```python
from build123d import *

# Parameters (mm, degrees)
CROQUIS1_W                                   = 70
CROQUIS1_H                                   = 30
SALIENTE_EXTRUIR1_DEPTH                      = 3
SALIENTE_EXTRUIR2_DEPTH                      = 24
CORTAR_EXTRUIR1_DEPTH                        = 70.000004
CROQUIS5_R                                   = 1.5
CORTAR_EXTRUIR2_DEPTH                        = 3
REFRENTADO_PARA_TORNILLO_TAP_N_CON_C_2_COUNT = 2
REFRENTADO_PARA_TORNILLO_TAP_N_CON_C_2_PITCH = 30
REFRENTADO_PARA_TORNILLO_TAP_N_CON_C_3_COUNT = 2
REFRENTADO_PARA_TORNILLO_TAP_N_CON_C_3_PITCH = 18.848076825
REFRENTADO_PARA_TORNILLO_TAP_N_CON_C_4_COUNT = 2
REFRENTADO_PARA_TORNILLO_TAP_N_CON_C_4_PITCH = 40.929817982
REDONDEO1_R                                  = 5


with BuildPart() as part:
    # Croquis1 → Saliente-Extruir1 (new body)
    with BuildSketch(Plane.XY):
        with Locations((5.076335878, 0.496183206)):
            Rectangle(CROQUIS1_W, CROQUIS1_H)
    extrude(amount=SALIENTE_EXTRUIR1_DEPTH)

    # Croquis3 → Saliente-Extruir2 (add)
    with BuildSketch(Plane.XY.offset(3)):
        Polygon((-29.923664122, 0.496183206), (40.076335878, 0.496183206), (40.076335878, -4.503816794), (40.076335878, -14.503816794), (36.076335878, -14.503816794), (36.076335878, -4.503816794), (18.076335878, -4.503816794), (18.076335878, -14.503816794), (14.076335878, -14.503816794), (14.076335878, -4.503816794), (-3.923664122, -4.503816794), (-3.923664122, -14.503816794), (-7.923664122, -14.503816794), (-7.923664122, -4.503816794), (-25.923664122, -4.503816794), (-25.923664122, -14.503816794), (-29.923664122, -14.503816794), (-29.923664122, -4.503816794), align=None)
    extrude(amount=SALIENTE_EXTRUIR2_DEPTH)

    # Croquis4 → Cortar-Extruir1 (cut)
    with BuildSketch(Plane.ZY.offset(29.923664122)):
        with BuildLine():
            Line((27, -14.503816794), (27, -4.503816794))
            ThreePointArc((27, -4.503816794), (14.366976751, -7.984560996), (3, -14.503816794))
            Line((3, -14.503816794), (27, -14.503816794))
        make_face()
    extrude(amount=-CORTAR_EXTRUIR1_DEPTH, mode=Mode.SUBTRACT)

    # Croquis5 → Cortar-Extruir2 (cut)
    with BuildSketch(Plane.XY.offset(3)):
        with Locations((-9.923664122, 7.996183206)):
            Circle(CROQUIS5_R)
        with Locations(Location((20.076335878, 7.996183206, 0), (0, 0, 180))):
            Circle(CROQUIS5_R)
        with Locations((-16.923664122, -9.503816794)):
            Circle(CROQUIS5_R)
        with Locations(Location((27.076335878, -9.503816794, 0), (0, 0, 180))):
            Circle(CROQUIS5_R)
    extrude(amount=-CORTAR_EXTRUIR2_DEPTH, mode=Mode.SUBTRACT)

    # Croquis7 → Refrentado para tornillo tapón con cabeza plana de clavija de M31 (revolve, cut)
    with BuildSketch(Plane(origin=(-9.923664122, 7.996183206, 3), x_dir=(0, -1, 0), z_dir=(1, 0, 0))):
        Polygon((0, 0), (0, 3), (1.7, 3), (1.7, 1.66), (3.36, 0), align=None)
    refrentado_para_tornillo_tap_n_con_cabez = revolve(axis=Axis((-9.923664122, 7.996183206, 9.35), (0, 0, -1)), mode=Mode.SUBTRACT)

    # Refrentado para tornillo tap_n con c 2: Refrentado para tornillo tapón con cabeza plana de clavija de M31 ×2
    with Locations(*[(i * REFRENTADO_PARA_TORNILLO_TAP_N_CON_C_2_PITCH, 0, 0) for i in range(1, REFRENTADO_PARA_TORNILLO_TAP_N_CON_C_2_COUNT)]):
        add(refrentado_para_tornillo_tap_n_con_cabez, mode=Mode.SUBTRACT)

    # Refrentado para tornillo tap_n con c 3: Refrentado para tornillo tapón con cabeza plana de clavija de M31 ×2
    with Locations(*[Vector(-0.3713906763541037, -0.9284766908852593, 0) * (i * REFRENTADO_PARA_TORNILLO_TAP_N_CON_C_3_PITCH) for i in range(1, REFRENTADO_PARA_TORNILLO_TAP_N_CON_C_3_COUNT)]):
        add(refrentado_para_tornillo_tap_n_con_cabez, mode=Mode.SUBTRACT)

    # Refrentado para tornillo tap_n con c 4: Refrentado para tornillo tapón con cabeza plana de clavija de M31 ×2
    with Locations(*[Vector(0.9039864290798859, -0.42756114888913443, 0) * (i * REFRENTADO_PARA_TORNILLO_TAP_N_CON_C_4_PITCH) for i in range(1, REFRENTADO_PARA_TORNILLO_TAP_N_CON_C_4_COUNT)]):
        add(refrentado_para_tornillo_tap_n_con_cabez, mode=Mode.SUBTRACT)

    # Redondeo1
    # the kernel refuses this fillet: 5 mm, written as the material it takes off along each edge
    with BuildSketch(Plane(origin=(40.076335878, -14.503816794, 15.5), x_dir=(0, 1, 0), z_dir=(0, 0, -1)), Plane(origin=(-29.923664122, -14.503816794, -12.5), x_dir=(0, 1, 0), z_dir=(0, 0, 1)), Plane(origin=(-29.923664122, 15.496183206, -12.5), x_dir=(1, 0, 0), z_dir=(0, 0, 1))) as redondeo1_piece_1:
        with BuildLine():
            CenterArc((REDONDEO1_R, -REDONDEO1_R), REDONDEO1_R, 90, 90)
            Line((0, -REDONDEO1_R), (0, 0))
            Line((0, 0), (REDONDEO1_R, 0))
        make_face()
    extrude(amount=28, mode=Mode.SUBTRACT)
    with BuildSketch(Plane(origin=(40.076335878, 15.496183206, -12.5), x_dir=(-1, 0, 0), z_dir=(0, 0, 1))) as redondeo1_piece_2:
        with BuildLine():
            CenterArc((REDONDEO1_R, REDONDEO1_R), REDONDEO1_R, 180, 90)
            Line((0, REDONDEO1_R), (0, 0))
            Line((0, 0), (REDONDEO1_R, 0))
        make_face()
    extrude(amount=28, mode=Mode.SUBTRACT)


solid = part.part
```
Verification items for the finished model (mm, model axes). A direction names the side the tool comes from. Coordinates: 2 decimals unless noted, no trailing zeros. Loops run counter-clockwise (first coordinate to the right, second up) from the corner with the lowest first, then second, coordinate; pieces in that order, holes last. Notation, with made-up numbers: (15.25, 55) -> (69.25, 55) arc R27 ccw to (69.25, 94) -> close; hole circle Ø8 at (-25.75, 10). An arc over 180 degrees is marked (long way). Put each result on its own line as item: value.
1. Mould release check, pull along Y, two halves, no side actions. Record for faces 4 (the face through (5, 15.496, 1)), 5 (the face through (14.076, -7, 9)), 6 (the face through (5, -14.504, 1)), 7 (the face through (28.736, -9.135, 0.679)): pulls with the +Y half, pulls with the -Y half, needs draft (parallel to the pull), parting line crosses it, or undercut.
Result set:
face 4: pulls with the +Y half
face 5: needs draft
face 6: pulls with the -Y half
face 7: undercut
2. Tool access check on faces 1 (the face through (5, 8, 3)), 2 (the face through (-29.05, -12.33, 2.99)), 3 (the face through (29, -6, 3)). Record the directions out of +Z, -Z, +X, -X, +Y, -Y that give a thin tool (end or side, any length) a straight path to the whole face; none if there is none.
Result set:
face 1: +Z, +X, -X, +Y
face 2: +Z, -Z, -X, -Y
face 3: +Z, -Y
3. Section check D-D, the plane y = 8.5. Give the number of separate pieces and of enclosed holes in the cut face, then the cut area to 3 significant figures.
Result set:
separate pieces: 3
enclosed holes: 0
area: 185 mm^2
4. Thickness scan on line 1 (Y direction, x = -11, z = 23); line 2 (Z direction, x = 7, y = -6); line 3 (Y direction, x = 15.5, z = 18.25). Record the ranges inside material, lowest first.
Result set:
line 1: y = -4.5 to 0.5
line 2: z = 0 to 3
line 3: y = -6.54 to 0.5
5. Gauge pin test, flat ends, axial feed: P1, Ø14.5, axis at x = 24, z = 12, coming from the -Y side; P2, Ø5.5, axis at x = 27.08, y = -9.5, coming from the +Z side; P3, Ø3, axis at x = -13.5, z = 18.5, coming from the +Y side. Record the tip position at first contact, or that the pin passes through.
Result set:
P1: stops at y = -11.27
P2: stops at z = 2.4
P3: stops at y = 0.5
6. Section check C-C, the plane y = 3.5. Record the boundary of the cut face in (x, z), then the cut area to 3 significant figures.
Result set:
outline: (-29.92, 0) -> (40.08, 0) -> (40.08, 3) -> (-29.92, 3) -> close
area: 210 mm^2
7. Section check B-B, the plane z = 6.5. Record the boundary of the cut face in (x, y).
Result set:
outline: (-29.92, -9.5) arc R5 ccw to (-29.21, -12.08) -> (-25.92, -12.08) -> (-25.92, -4.5) -> (-7.92, -4.5) -> (-7.92, -12.08) -> (-3.92, -12.08) -> (-3.92, -4.5) -> (14.08, -4.5) -> (14.08, -12.08) -> (18.08, -12.08) -> (18.08, -4.5) -> (36.08, -4.5) -> (36.08, -12.08) -> (39.36, -12.08) arc R5 ccw to (40.08, -9.5) -> (40.08, 0.5) -> (-29.92, 0.5) -> close
8. Section check A-A, the plane x = 0.5. Record the boundary of the cut face in (y, z), then the cut area to 3 significant figures.
Result set:
outline: (-14.5, 0) -> (15.5, 0) -> (15.5, 3) -> (0.5, 3) -> (0.5, 27) -> (-4.5, 27) -> (-4.5, 3) -> (-14.5, 3) -> close
area: 210 mm^2
